Answer from the drawing. Dimensions are ordinates in mm from the lowest x, y and z of the part. A direction names the side the tool comes from. Coordinates: 2 decimals unless noted, no trailing zeros. Order: outer loops, then holes, each group sorted by start corner. A loop starts at its lowest first (then second) coordinate and runs counter-clockwise, first axis right, second up. Notation, with made-up numbers: (-24, 0) - (33, 0) arc R26 cw to (33, 33) - close; hole circle Ø8 at (43.25, -4.75). An arc over 180 degrees is marked (long way). Use a Markdown table: item, result. Add a question column.
Item 1: The mould has two halves that part along X. Classify the marked faces 1, 2 and 3: released by +X, released by -X, zero draft, split by the parting line, or undercut.
Item 2: The part is cut by section C-C, the plane y = 9.5. Give the vertices of the cut face in (x, z), then the cut area to 3 significant figures.
Item 3: Find the intervals of material crossed by line 1 along Y through (x, z) = (7.9, 2.7); line 2 along Y through (x, z) = (10.15, 2.65); line 3 along Y through (x, z) = (2.25, 0.5), in increasing order.
Item 4: The part is cut by section D-D, the plane x = 10.15. Give the vertices of the cut face in (y, z).
Item 5: For the marked faces 4 and 5, determine the directions among +Z, -Z, +X, -X, +Y, -Y from which every point of the face is accessible in a straight line to the end or side of a thin tool.
Item 6: The part is cut by section B-B, the plane x = 7.9. Give the vertices of the cut face in (y, z), then the cut area to 3 significant figures.
Item 7: The part is cut by section A-A, the plane z = 1.15. Give the vertices of the cut face in (x, y), then the cut area to 3 significant figures.
Item 8: A flat-ended cylindrical pin translates along its axis: P1, Ø1.1, axis at y = 3.5, z = 3.5, coming from the -X side. Find the tip coordinate at first contact, or state that the pin passes through.
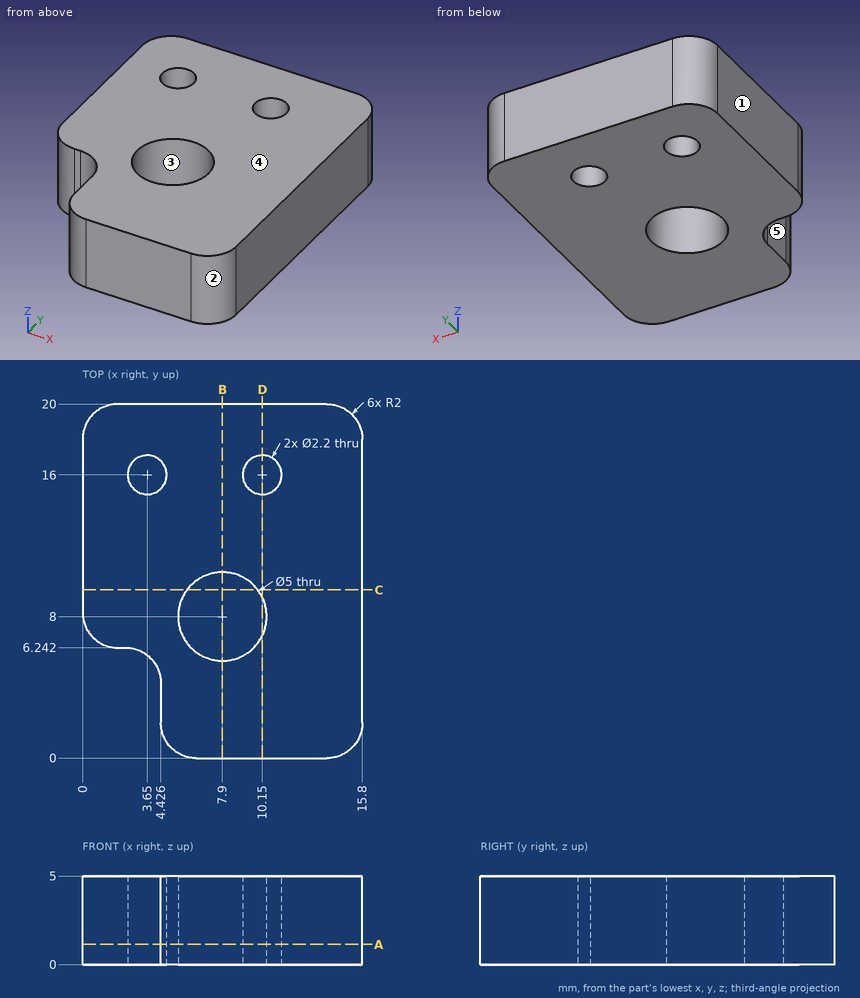
Solution:
| question | item | result |
|---|---|---|
| 1 | face 1 | released by -X |
| 1 | face 2 | released by +X |
| 1 | face 3 | undercut |
| 2 | outline | (0, 0) - (5.9, 0) - (5.9, 5) - (0, 5) - close; (9.9, 0) - (15.8, 0) - (15.8, 5) - (9.9, 5) - close |
| 2 | area | 59.0 mm2 |
| 3 | line 1 | y = 0 to 5.5, 10.5 to 20 |
| 3 | line 2 | y = 0 to 6.91, 9.09 to 14.9, 17.1 to 20 |
| 3 | line 3 | y = 6.24 to 20 |
| 4 | outline | (0, 0) - (6.91, 0) - (6.91, 5) - (0, 5) - close; (9.09, 0) - (14.9, 0) - (14.9, 5) - (9.09, 5) - close; (17.1, 0) - (20, 0) - (20, 5) - (17.1, 5) - close |
| 5 | face 4 | +Z, +X, -X, +Y, -Y |
| 5 | face 5 | +Z, -Z, -X, -Y |
| 6 | outline | (0, 0) - (5.5, 0) - (5.5, 5) - (0, 5) - close; (10.5, 0) - (20, 0) - (20, 5) - (10.5, 5) - close |
| 6 | area | 75.0 mm2 |
| 7 | outline | (0, 8.24) arc R2 ccw to (2, 6.24) - (2.43, 6.24) arc R2 cw to (4.43, 4.24) - (4.43, 2) arc R2 ccw to (6.43, 0) - (13.8, 0) arc R2 ccw to (15.8, 2) - (15.8, 18) arc R2 ccw to (13.8, 20) - (2, 20) arc R2 ccw to (0, 18) - close; hole circle Ø2.2 at (3.65, 16); hole circle Ø5 at (7.9, 8); hole circle Ø2.2 at (10.15, 16) |
| 7 | area | 258 mm2 |
| 8 | P1 | stops at x = 4.43 |
